Geometry: final body of the model. Coordinates: model frame, mm. Coordinates: 2 decimals unless noted, no trailing zeros. Write each loop counter-clockwise with the first axis right and the second up, starting at its lowest first coordinate (ties: lowest second). Pieces come first, ordered by that corner, then holes. Notation, with made-up numbers: M 17.25,-23 L 23.25,-23 A19 ccw 23.25,4 Z; hole C 31,41.25 d1. An arc over 180 degrees is marked long. Write item = value, one per line. Start each with the question number.
Item 1: Section C-C on y = 18. Output: boundary loops of the cut face in (x, z), plus the area to 3 significant figures.
Item 2: Ray query, L1, parallel to Y at x = -66.4, z = 1.9; L2, parallel to Y at x = 38.1, z = 0.7; L3, parallel to X at y = 16.5, z = 2.35. Return the intervals inside material, ascending. Write a range as [from, to].
Item 3: Pull-direction query (X, two-part tool) for faces 1 (the cylindrical face through (-68.63, 26.89, 1.5)), 2 (the cylindrical face through (-68.63, -20.11, 1.5)), 3 (the flat face through (-2, 1, 3.048)); classes: +X half, -X half, draft (parallel to the pull), parting line (faces both ways), or undercut.
Item 4: Section D-D on z = 0.55. Give the number of separate pieces and of enclosed holes in the cut face, plus the area to 3 significant figures.
Item 5: Section A-A on x = -66.4. Output: boundary loops of the cut face in (y, z), plus the area to 3 significant figures.
Item 6: Section B-B on y = -20.4. Output: boundary loops of the cut face in (x, z).
Autodesk Inventor part; units mm, degrees
ref_plane "YZ Plane" through (0, 0, 0) normal (1, 0, 0) x (0, 1, 0)
ref_plane "XZ Plane" through (0, 0, 0) normal (0, 1, 0) x (-1, 0, 0)
ref_plane "XY Plane" through (0, 0, 0) normal (0, 0, 1) x (1, 0, 0)
sketch "Sketch1" plane through (0, 0, 0) normal (0, 0, 1) x (1, 0, 0)
  line L0 (114.3, 63.5) -> (-114.3, 63.5)
  line L1 (-114.3, 63.5) -> (-114.3, -63.5)
  line L2 (-114.3, -63.5) -> (114.3, -63.5)
  line L3 (114.3, -63.5) -> (114.3, 63.5)
  point P0 (0, 0)
  dimension "d0" = 228.6
  dimension "d1" = 127
extrude "Plate1" add sketch "Sketch1" along normal blind 3.048
sketch "Sketch2" plane through (0, 0, 3.048) normal (0, 0, 1) x (1, 0, 0)
  line L0 (-114.3, 63.5) -> (-114.3, -63.5)
  line L1 (-114.3, -63.5) -> (-114.3, -60.325)
  line L2 (-114.3, -60.325) -> (-76.2, -60.325)
  line L3 (-76.2, -60.325) -> (-38.1, -60.325)
  line L4 (-38.1, -60.325) -> (0, -60.325)
  line L5 (0, -60.325) -> (38.1, -60.325)
  line L6 (38.1, -60.325) -> (76.2, -60.325)
  line L7 (76.2, -60.325) -> (114.3, -60.325)
  line L8 (114.3, -63.5) -> (114.3, 63.5)
  point P0 (0, 0)
  dimension "d3" = 3.175
  dimension "d4" = 38.1
  dimension "d5" = 38.1
  dimension "d6" = 38.1
  dimension "d7" = 38.1
hole "Hole1" at (-76.2, -60.325, 3.048) at (-38.1, -60.325, 3.048) at (0, -60.325, 3.048) at (38.1, -60.325, 3.048) at (76.2, -60.325, 3.048) direction (0, 0, -1) diameter 3.2766 depth 3.048
sketch "Sketch3" plane through (0, 0, 3.048) normal (0, 0, 1) x (1, 0, 0)
  line L0 (-114.3, -63.5) -> (114.3, -63.5)
  line L1 (-114.3, -63.5) -> (-114.3, -25.4)
  line L2 (-114.3, -63.5) -> (-114.3, 63.5)
  line L3 (-114.3, -25.4) -> (-88.9, -25.4)
  line L4 (-88.9, -25.4) -> (-88.9, 31.6)
  line L5 (-88.9, 31.6) -> (-43.9, 31.6)
  line L6 (-43.9, 31.6) -> (-43.9, -25.4)
  line L7 (-43.9, -25.4) -> (-88.9, -25.4)
  line L8 (-66.4, -25.4) -> (-66.4, -20.4)
  line L9 (-66.4, 31.6) -> (-66.4, 26.6)
  line L10 (-43.9, 31.6) -> (-36.28, 31.6)
  line L11 (-36.28, 31.6) -> (-36.28, -25.4)
  line L12 (-36.28, -25.4) -> (8.72, -25.4)
  line L13 (8.72, -25.4) -> (8.72, 31.6)
  line L14 (8.72, 31.6) -> (-36.28, 31.6)
  line L15 (-13.78, 31.6) -> (-13.78, 26.6)
  line L16 (-13.78, -25.4) -> (-13.78, -20.4)
  point P0 (0, 0)
  dimension "d15" = 38.1
  dimension "d16" = 25.4
  dimension "d17" = 57
  dimension "d18" = 45
  dimension "d19" = 5
  dimension "d20" = 5
  dimension "d21" = 7.62
  dimension "d22" = 45
  dimension "d23" = 5
  dimension "d24" = 5
hole "Hole2" at (-66.4, 26.6, 3.048) at (-13.78, 26.6, 3.048) at (-13.78, -20.4, 3.048) at (-66.4, -20.4, 3.048) direction (0, 0, -1) diameter 4.4958 depth 3.048
sketch "Sketch4" plane through (0, 0, 3.048) normal (0, 0, 1) x (1, 0, 0)
  line L0 (-114.3, -63.5) -> (114.3, -63.5)
  line L1 (114.3, -63.5) -> (114.3, -25.4)
  line L2 (114.3, -63.5) -> (114.3, 63.5)
  line L3 (114.3, -25.4) -> (88.9, -25.4)
  line L4 (88.9, -25.4) -> (88.9, -2.794)
  line L5 (88.9, -2.794) -> (76.2, -2.794)
  line L6 (76.2, -2.794) -> (71.12, -2.794)
  line L7 (71.12, -2.794) -> (58.42, -2.794)
  line L8 (58.42, -2.794) -> (53.34, -2.794)
  line L9 (53.34, -2.794) -> (40.64, -2.794)
  line L10 (40.64, -2.794) -> (40.64, -25.4)
  line L11 (40.64, -25.4) -> (53.34, -25.4)
  line L12 (53.34, -25.4) -> (53.34, -2.794)
  line L13 (58.42, -2.794) -> (58.42, -25.4)
  line L14 (58.42, -25.4) -> (71.12, -25.4)
  line L15 (71.12, -25.4) -> (71.12, -2.794)
  line L16 (76.2, -2.794) -> (76.2, -25.4)
  line L17 (76.2, -25.4) -> (88.9, -25.4)
  point P0 (0, 0)
  dimension "d32" = 38.1
  dimension "d33" = 25.4
  dimension "d34" = 22.606
  dimension "d35" = 12.7
  dimension "d36" = 5.08
  dimension "d37" = 12.7
  dimension "d38" = 5.08
  dimension "d39" = 12.7
extrude "Cut1" cut sketch "Sketch4" against normal blind 3.048
sketch "Sketch5" plane through (0, 0, 3.048) normal (0, 0, 1) x (1, 0, 0)
  line L0 (-114.3, -63.5) -> (114.3, -63.5)
  line L1 (114.3, -63.5) -> (114.3, 12.7)
  line L2 (114.3, -63.5) -> (114.3, 63.5)
  line L3 (114.3, 12.7) -> (88.9, 12.7)
  line L4 (88.9, 12.7) -> (80.518, 12.7)
  line L5 (80.518, 12.7) -> (80.518, 29.718)
  line L6 (80.518, 29.718) -> (74.168, 29.718)
  line L7 (74.168, 29.718) -> (74.168, 12.7)
  line L8 (74.168, 12.7) -> (65.786, 12.7)
  line L9 (65.786, 12.7) -> (65.786, 29.718)
  line L10 (65.786, 29.718) -> (74.168, 29.718)
  line L11 (80.518, 29.718) -> (88.9, 29.718)
  line L12 (88.9, 29.718) -> (88.9, 12.7)
  line L13 (65.786, 29.718) -> (59.436, 29.718)
  line L14 (59.436, 29.718) -> (59.436, 12.7)
  line L15 (59.436, 12.7) -> (51.054, 12.7)
  line L16 (51.054, 12.7) -> (51.054, 29.718)
  line L17 (51.054, 29.718) -> (59.436, 29.718)
  line L18 (51.054, 29.718) -> (44.704, 29.718)
  line L19 (44.704, 29.718) -> (44.704, 12.7)
  line L20 (44.704, 12.7) -> (36.322, 12.7)
  line L21 (36.322, 12.7) -> (36.322, 29.718)
  line L22 (36.322, 29.718) -> (44.704, 29.718)
  point P0 (0, 0)
  dimension "d42" = 76.2
  dimension "d43" = 25.4
  dimension "d44" = 270
  dimension "d45" = 8.382
  dimension "d46" = 17.018
  dimension "d47" = 6.35
  dimension "d48" = 8.382
  dimension "d49" = 6.35
  dimension "d50" = 8.382
  dimension "d51" = 6.35
  dimension "d52" = 8.382
extrude "Cut2" cut sketch "Sketch5" against normal blind 3.048
sketch "Sketch6" plane through (0, 0, 3.048) normal (0, 0, 1) x (1, 0, 0)
  line L0 (-114.3, 63.5) -> (114.3, 63.5)
  line L1 (-114.3, 63.5) -> (-114.3, 50.8)
  line L2 (-114.3, 63.5) -> (-114.3, -63.5)
  line L3 (-114.3, 50.8) -> (-38.1, 50.8)
  line L4 (-38.1, 50.8) -> (38.1, 50.8)
  line L5 (38.1, 50.8) -> (114.246, 50.8)
  point P0 (0, 0)
  dimension "d55" = 12.7
  dimension "d56" = 76.2
  dimension "d57" = 76.2
hole "Hole3" at (-38.1, 50.8, 3.048) at (38.1, 50.8, 3.048) direction (0, 0, -1) diameter 2.1565 depth 8.8646
sketch "Sketch7" plane through (0, 0, 0) normal (0, 0, -1) x (-1, 0, 0)
  circle A0 centre (38.1, 50.8) radius 1.0782
  circle A1 centre (-38.1, 50.8) radius 1.0782
  line L0 (-65.786, 29.718) -> (-65.786, 12.7)
  line L1 (-65.786, 12.7) -> (-74.168, 12.7)
  line L2 (-74.168, 12.7) -> (-74.168, 29.718)
  line L3 (-74.168, 29.718) -> (-65.786, 29.718)
  line L4 (-36.322, 29.718) -> (-36.322, 12.7)
  line L5 (-36.322, 12.7) -> (-44.704, 12.7)
  line L6 (-44.704, 12.7) -> (-44.704, 29.718)
  line L7 (-44.704, 29.718) -> (-36.322, 29.718)
  line L8 (-51.054, 29.718) -> (-51.054, 12.7)
  line L9 (-51.054, 12.7) -> (-59.436, 12.7)
  line L10 (-59.436, 12.7) -> (-59.436, 29.718)
  line L11 (-59.436, 29.718) -> (-51.054, 29.718)
  line L12 (-88.9, 29.718) -> (-80.518, 29.718)
  line L13 (-80.518, 29.718) -> (-80.518, 12.7)
  line L14 (-80.518, 12.7) -> (-88.9, 12.7)
  line L15 (-88.9, 12.7) -> (-88.9, 29.718)
  line L16 (-58.42, -2.794) -> (-58.42, -25.4)
  line L17 (-58.42, -25.4) -> (-71.12, -25.4)
  line L18 (-71.12, -25.4) -> (-71.12, -2.794)
  line L19 (-71.12, -2.794) -> (-58.42, -2.794)
  line L20 (-40.64, -2.794) -> (-40.64, -25.4)
  line L21 (-40.64, -25.4) -> (-53.34, -25.4)
  line L22 (-53.34, -25.4) -> (-53.34, -2.794)
  line L23 (-53.34, -2.794) -> (-40.64, -2.794)
  line L24 (-88.9, -2.794) -> (-76.2, -2.794)
  line L25 (-76.2, -2.794) -> (-76.2, -25.4)
  line L26 (-76.2, -25.4) -> (-88.9, -25.4)
  line L27 (-88.9, -25.4) -> (-88.9, -2.794)
  circle A2 centre (13.78, -20.4) radius 2.2479
  circle A3 centre (66.4, 26.6) radius 2.2479
  circle A4 centre (13.78, 26.6) radius 2.2479
  circle A5 centre (66.4, -20.4) radius 2.2479
  circle A6 centre (-38.1, -60.325) radius 1.6383
  circle A7 centre (38.1, -60.325) radius 1.6383
  circle A8 centre (76.2, -60.325) radius 1.6383
  circle A9 centre (0, -60.325) radius 1.6383
  circle A10 centre (-76.2, -60.325) radius 1.6383
  line L28 (-114.3, 63.5) -> (114.3, 63.5)
  line L29 (-114.3, -63.5) -> (-114.3, 63.5)
  line L30 (114.3, -63.5) -> (-114.3, -63.5)
  line L31 (114.3, 63.5) -> (114.3, -63.5)
  point P0 (0, 0)
hole "Hole4" at (40.64, -2.794, 0) at (40.64, -25.4, 0) at (53.34, -25.4, 0) at (53.34, -2.794, 0) at (58.42, -2.794, 0) at (58.42, -25.4, 0) at (71.12, -25.4, 0) at (71.12, -2.794, 0) at (76.2, -2.794, 0) at (76.2, -25.4, 0) at (88.9, -25.4, 0) at (88.9, -2.794, 0) at (80.518, 29.718, 0) at (88.9, 29.718, 0) at (88.9, 12.7, 0) at (80.518, 12.7, 0) at (74.168, 12.7, 0) at (74.168, 29.718, 0) at (65.786, 29.718, 0) at (65.786, 12.7, 0) at (59.436, 12.7, 0) at (59.436, 29.718, 0) at (51.054, 29.718, 0) at (51.054, 12.7, 0) at (44.704, 12.7, 0) at (36.322, 12.7, 0) at (36.322, 29.718, 0) at (44.704, 29.718, 0) direction (0, 0, 1) diameter 2.794 depth 3.048
sketch "Sketch8" plane through (0, 0, 3.048) normal (0, 0, 1) x (1, 0, 0)
  line L0 (-114.3, -63.5) -> (114.3, -63.5)
  line L1 (114.3, -63.5) -> (63.5, -63.5)
  line L2 (63.5, -63.5) -> (63.5, -38.1)
  line L3 (63.5, -38.1) -> (38.1, -38.1)
  line L4 (38.1, -38.1) -> (12.7, -38.1)
  point P0 (0, 0)
  dimension "d72" = 50.8
  dimension "d73" = 25.4
  dimension "d74" = 25.4
  dimension "d75" = 25.4
hole "Hole5" at (38.1, -38.1, 3.048) direction (0, 0, -1) diameter 6.7564 depth 3.048
equation "\"d13\" = Thickness"
equation "\"d30\" = Thickness"
equation "\"d40\" = Thickness"
equation "\"d53\" = Thickness"
equation "\"d70\" = Thickness"
equation "\"d81\" = Thickness"
equation "\"d2\" = Thickness"
equation "\"BendRadius\" = Thickness"
equation "\"BendReliefWidth\" = Thickness"
equation "\"BendReliefDepth\" = 0.5 * Thickness"
equation "\"CornerReliefSize\" = 4 * Thickness"
equation "\"MinimumRemnant\" = 2 * Thickness"
equation "\"TransitionRadius\" = BendRadius"
equation "\"JacobiRadiusSize\" = BendRadius"
equation "\"GapSize\" = Thickness"
properties part number "sheetmetalleft2.0"
Responses:
q1.outline = M -114.3,0 L 36.32,0 L 36.32,3.05 L -114.3,3.05 Z; M 44.7,0 L 51.05,0 L 51.05,3.05 L 44.7,3.05 Z; M 59.44,0 L 65.79,0 L 65.79,3.05 L 59.44,3.05 Z; M 74.17,0 L 80.52,0 L 80.52,3.05 L 74.17,3.05 Z; M 88.9,0 L 114.3,0 L 114.3,3.05 L 88.9,3.05 Z
q1.area = 595 mm²
q2.L1 = [-63.5, -22.65], [-18.15, 24.35], [28.85, 63.5]
q2.L2 = [-63.5, -61.96], [-58.69, -41.48], [-34.72, 12.7], [29.72, 49.72], [51.88, 63.5]
q2.L3 = [-114.3, 36.32], [44.7, 51.05], [59.44, 65.79], [74.17, 80.52], [88.9, 114.3]
q3.face_1 = undercut
q3.face_2 = undercut
q3.face_3 = draft
q4.separate_pieces = 1
q4.enclosed_holes = 19
q4.area = 27,300 mm²
q5.outline = M -63.5,0 L -22.65,0 L -22.65,3.05 L -63.5,3.05 Z; M -18.15,0 L 24.35,0 L 24.35,3.05 L -18.15,3.05 Z; M 28.85,0 L 63.5,0 L 63.5,3.05 L 28.85,3.05 Z
q5.area = 360 mm²
q6.outline = M -114.3,0 L -68.65,0 L -68.65,3.05 L -114.3,3.05 Z; M -64.15,0 L -16.03,0 L -16.03,3.05 L -64.15,3.05 Z; M -11.53,0 L 40.64,0 L 40.64,3.05 L -11.53,3.05 Z; M 53.34,0 L 58.42,0 L 58.42,3.05 L 53.34,3.05 Z; M 71.12,0 L 76.2,0 L 76.2,3.05 L 71.12,3.05 Z; M 88.9,0 L 114.3,0 L 114.3,3.05 L 88.9,3.05 Z
